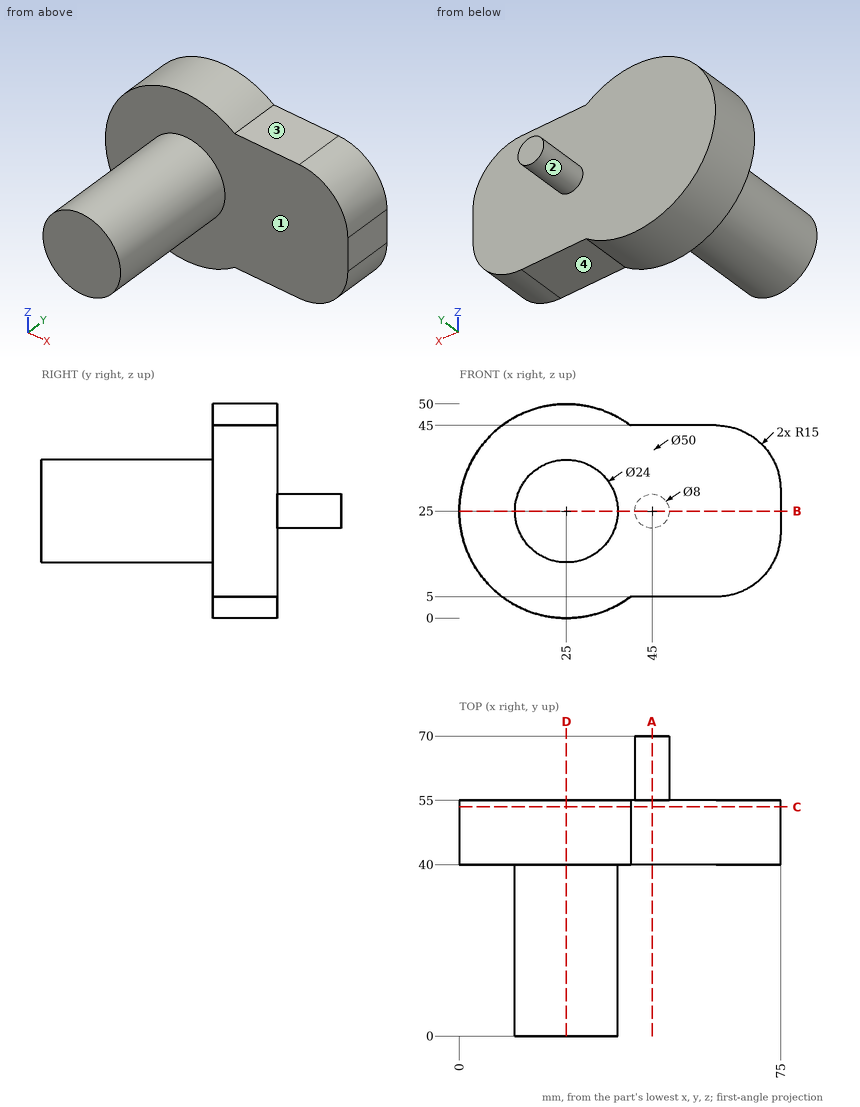
Job drawing, mm, ordinate dimensions from the low corner. One solid piece. A direction names the side the tool comes from. Coordinates: 2 decimals unless noted, no trailing zeros. Order: outer loops, then holes, each group sorted by start corner. A loop starts at its lowest first (then second) coordinate and runs counter-clockwise, first axis right, second up. Notation, with made-up numbers: M 88,-28 L 143,-28 A19 ccw 143,-7 Z; hole C 42,-39.75 d6. An arc over 180 degrees is marked long. Return JSON: item names as keys, results as strings.
1. Flat gauge pins, fed straight in: pin 1 (4.5 mm diameter, centred on x = 53.5, y = 49, fed in from -Z); pin 2 (2 mm diameter, centred on y = 14, z = 19, fed in from +X); pin 3 (8 mm diameter, centred on x = 53.5, y = 52.5, fed in from +Z). Where does each tip first touch, or does it go through?
Ans:
{"pin 1": "z = 5", "pin 2": "x = 35.91", "pin 3": "z = 45"}
2. Drill centre lines: probe 1 along Y at (x, z) = (64, 18); probe 2 along Y at (x, z) = (21, 27); probe 3 along Z at (x, y) = (48, 50.5). Where is each one in solid material? Low to high.
Ans:
{"probe 1": "40 to 55", "probe 2": "0 to 55", "probe 3": "5 to 45"}
3. Saw through at D-D (x = 25). Give the cut face in (y, z), and give its area (3 significant figures).
Ans:
{"outline": "M 0,13 L 40,13 L 40,0 L 55,0 L 55,50 L 40,50 L 40,37 L 0,37 Z", "area": "1,710 mm^2"}
4. Saw through at C-C (y = 53.5). Give the cut face in (x, z), and give its area (3 significant figures).
Ans:
{"outline": "M 40,5 L 60,5 A15 ccw 75,20 L 75,30 A15 ccw 60,45 L 40,45 A25 ccw long Z", "area": "2,990 mm^2"}
5. Saw through at A-A (x = 45). Give the cut face in (y, z), and give its area (3 significant figures).
Ans:
{"outline": "M 40,5 L 55,5 L 55,21 L 70,21 L 70,29 L 55,29 L 55,45 L 40,45 Z", "area": "720 mm^2"}
6. Tool access for the marked faces 1, 2, 3 and 4: list every direction of +Z, -Z, +X, -X, +Y, -Y with a clear straight run to the whole face (end or side of a thin tool).
Ans:
{"face 1": "-Y", "face 2": "+Y", "face 3": "+Z, +X, +Y, -Y", "face 4": "-Z, +X, +Y, -Y"}
7. Saw through at B-B (z = 25). Give the cut face in (x, y).
Ans:
{"outline": "M 0,40 L 13,40 L 13,0 L 37,0 L 37,40 L 75,40 L 75,55 L 49,55 L 49,70 L 41,70 L 41,55 L 0,55 Z"}
